```python
from build123d import *

# Parameters (mm, degrees)
SKETCH1_R           = 12.192
BOSS_EXTRUDE1_DEPTH = 46.99
SKETCH2_R           = 12.4587
BOSS_EXTRUDE2_DEPTH = 27.94
SKETCH3_R           = 3.4925
BOSS_EXTRUDE3_DEPTH = 2.54
SKETCH4_R           = 1.9939
BOSS_EXTRUDE4_DEPTH = 10.9982
FILLET1_R           = 0.635
FILLET2_R           = 0.635
SKETCH5_R           = 1.0033
CUT_EXTRUDE1_DEPTH  = 12.7


with BuildPart() as part:
    # Sketch1 → Boss-Extrude1 (new body)
    with BuildSketch(Plane(origin=(0, 0, 0), x_dir=(1, 0, 0), z_dir=(0, 1, 0))):
        with Locations(Location((0, 0, 0), (0, 0, 270))):
            Circle(SKETCH1_R)
    extrude(amount=BOSS_EXTRUDE1_DEPTH)

    # Sketch2 → Boss-Extrude2 (add)
    with BuildSketch(Plane(origin=(0, 46.99, 0), x_dir=(1, 0, 0), z_dir=(0, 1, 0))):
        with Locations(Location((0, 0, 0), (0, 0, 270))):
            Circle(SKETCH2_R)
    extrude(amount=BOSS_EXTRUDE2_DEPTH)

    # Sketch3 → Boss-Extrude3 (add)
    with BuildSketch(Plane(origin=(0, 74.93, 0), x_dir=(1, 0, 0), z_dir=(0, 1, 0))):
        with Locations(Location((0, 0, 0), (0, 0, 270))):
            Circle(SKETCH3_R)
    extrude(amount=BOSS_EXTRUDE3_DEPTH)

    # Sketch4 → Boss-Extrude4 (add)
    with BuildSketch(Plane(origin=(0, 77.47, 0), x_dir=(1, 0, 0), z_dir=(0, 1, 0))):
        with Locations(Location((0, 0, 0), (0, 0, 270))):
            Circle(SKETCH4_R)
    extrude(amount=BOSS_EXTRUDE4_DEPTH)

    # Fillet1
    fillet1_edges = [part.edges().sort_by_distance(p)[0] for p in [
        (0, 0, -12.192),
        (0, 74.93, -12.4587),
    ]]
    fillet(fillet1_edges, radius=FILLET1_R)

    # Fillet2
    fillet2_edges = [part.edges().sort_by_distance(p)[0] for p in [
        (0, 77.47, -3.4925),
    ]]
    fillet(fillet2_edges, radius=FILLET2_R)

    # Sketch5 → Cut-Extrude1 (cut)
    with BuildSketch(Plane(origin=(0, 74.93, 0), x_dir=(1, 0, 0), z_dir=(0, 1, 0))):
        with Locations(Location((7.62, 0, 0), (0, 0, 270))):
            Circle(SKETCH5_R)
        with Locations(Location((-7.62, 0, 0), (0, 0, 90))):
            Circle(SKETCH5_R)
    extrude(amount=-CUT_EXTRUDE1_DEPTH, mode=Mode.SUBTRACT)


solid = part.part
```
Can you work these out from the model? Positions are in its coordinate system, mm. A direction names the side the tool comes from. Round coordinates to 2 decimals unless told otherwise and drop trailing zeros. Loops run counter-clockwise (first coordinate to the right, second up) from the corner with the lowest first, then second, coordinate; pieces in that order, holes last.
Item 1: Suppose I cut it at C-C, the plane y = 52. Write out the boundary of the cut face in (x, z).
Item 2: Which directions (+Z, -Z, +X, -X, +Y, -Y) give clear straight access to the entire face, cutting with the end or side of a thin tool? Please do faces 4 (the flat face through (0, 0, 0)), 5 (the cylindrical face through (10.28, 23.488, 6.554)), 6 (the flat face through (-2.5, 74.93, -2.8)).
Item 3: Please list where these lines run through material, in increasing order: L1, parallel to X at y = 71.5, z = 0; L2, parallel to Y at x = -10.75, z = -0.75; L3, parallel to Y at x = -0.25, z = 3.
Item 4: If we mould it in two halves opening along X, with no side actions, what happens to faces 1 (the cylindrical face through (3.463, 75.869, -0.455)), 2 (the cylindrical face through (8.615, 68.669, -0.131)), 3 (the flat face through (0, 88.468, 0))? For each: +X half, -X half, draft (parallel to the pull), parting line (faces both ways), or undercut.
Item 5: Suppose I cut it at B-B, the plane y = 10. Write out the boundary of the cut face in (x, z).
Item 6: Will these pins go through, and if not, where does the flat tip stop? pin 1 Ø1.5 at (y, z) = (64.5, 1.5) entering from -X; pin 2 Ø10 at (x, z) = (1.5, 3.5) entering from -Y; pin 3 Ø2.5 at (x, z) = (-7.62, 0) entering from +Y; pin 4 Ø6 at (y, z) = (50.5, -5) entering from -X.
Reported:
1. outline: circle Ø24.92 at (0, 0)
2. face 4: +Z, -Z, +X, -X, -Y
2. face 5: -Y
2. face 6: +Y
3. L1: x = -12.46 to -8.62, -6.62 to 6.62, 8.62 to 12.46
3. L2: y = 0 to 74.93
3. L3: y = 0 to 77.45
4. face 1: parting line
4. face 2: undercut
4. face 3: draft
5. outline: circle Ø24.38 at (0, 0)
6. pin 1: stops at x = -12.44
6. pin 2: stops at y = 0
6. pin 3: stops at y = 74.93
6. pin 4: stops at x = -12.3
